```python
from build123d import *

# Parameters (mm, degrees)
SKETCH1_W                      = 76.2
SKETCH1_H                      = 66.04
BOSS_EXTRUDE1_DEPTH            = 20.32
SKETCH2_R                      = 3.749999993
CUT_EXTRUDE1_DEPTH             = 57.15
SKETCH4_W                      = 8
SKETCH4_H                      = 8
CUT_EXTRUDE4_DEPTH             = 5.08
FILLET2_R                      = 2.54
SKETCH5_W                      = 50.8
SKETCH5_H                      = 66.04
BOSS_EXTRUDE2_DEPTH            = 2.54
BOSS_EXTRUDE3_DEPTH            = 25.4
SKETCH3_W                      = 14
SKETCH3_H                      = 7
CUT_EXTRUDE5_DEPTH             = 73.66
CUT_EXTRUDE5_DIRECTION_2_REACH = 29.94
SKETCH7_R                      = 6.35
BOSS_EXTRUDE4_DEPTH            = 30.48


with BuildPart() as part:
    # Sketch1 → Boss-Extrude1 (new body)
    with BuildSketch(Plane.XY):
        with Locations((38.1, 33.02)):
            Rectangle(SKETCH1_W, SKETCH1_H)
    extrude(amount=BOSS_EXTRUDE1_DEPTH)

    # Sketch2 → Cut-Extrude1 (cut)
    with BuildSketch(Plane(origin=(0, 66.04, 0), x_dir=(1, 0, 0), z_dir=(0, 1, 0))):
        with Locations(Location((17.78, -10.16, 0), (0, 0, 270))):  # turned: the seam where the file's is
            Circle(SKETCH2_R)
    extrude(amount=-CUT_EXTRUDE1_DEPTH, mode=Mode.SUBTRACT)

    # Sketch4 → Cut-Extrude4 (cut)
    with BuildSketch(Plane(origin=(0, 0, 0), x_dir=(-1, 0, 0), z_dir=(0, -1, 0))):
        with Locations((-10.16, -10.16)):
            Rectangle(SKETCH4_W, SKETCH4_H)
    extrude(amount=-CUT_EXTRUDE4_DEPTH, mode=Mode.SUBTRACT)

    # Fillet2
    fillet2_edges = [part.edges().sort_by_distance(p)[0] for p in [
        (17.78, 66.04, 6.410000007),
    ]]
    fillet(fillet2_edges, radius=FILLET2_R)

    # Sketch5 → Boss-Extrude2 (add)
    with BuildSketch(Plane(origin=(76.2, 0, 0), x_dir=(0, 0, -1), z_dir=(1, 0, 0))):
        with Locations((0, 33.02)):
            Rectangle(SKETCH5_W, SKETCH5_H)
    extrude(amount=BOSS_EXTRUDE2_DEPTH)

    # Sketch6 → Boss-Extrude3 (add)
    with BuildSketch(Plane(origin=(78.74, 0, 0), x_dir=(0, 0, -1), z_dir=(1, 0, 0))):
        Polygon((-25.4, 0), (-19.631407878, 0), (15.24, 0), (25.4, 0), (25.4, 63.5), (22.86, 63.5), (22.86, 2.54), (-22.86, 2.54), (-22.86, 63.5), (-25.4, 63.5), align=None)
    extrude(amount=BOSS_EXTRUDE3_DEPTH)

    # Sketch3 → Cut-Extrude5 (cut)
    with BuildSketch(Plane(origin=(76.2, 0, 0), x_dir=(0, 0, -1), z_dir=(1, 0, 0))):
        with Locations((-10.16, 8.58)):
            Rectangle(SKETCH3_W, SKETCH3_H)
    extrude(amount=-CUT_EXTRUDE5_DEPTH, mode=Mode.SUBTRACT)

    # Sketch3 → Cut-Extrude5 direction 2 (cut, up to next)
    with BuildSketch(Plane(origin=(76.2, 0, 0), x_dir=(0, 0, -1), z_dir=(1, 0, 0)), mode=Mode.PRIVATE) as cut_extrude5_direction_2_sk1:
        with Locations((-10.16, 8.58)):
            Rectangle(SKETCH3_W, SKETCH3_H)
    cut_extrude5_direction_2_tool1 = extrude(cut_extrude5_direction_2_sk1.sketch, amount=CUT_EXTRUDE5_DIRECTION_2_REACH, mode=Mode.PRIVATE) & part.part
    add(cut_extrude5_direction_2_tool1.solids().sort_by_distance((76.2, 8.58, 10.16))[0], mode=Mode.SUBTRACT)

    # Sketch7 → Boss-Extrude4 (add)
    with BuildSketch(Plane(origin=(0, 0, 0), x_dir=(-1, 0, 0), z_dir=(0, -1, 0))):
        with Locations(Location((-63.5, -10.16, 0), (0, 0, 270))):  # turned: the seam where the file's is
            Circle(SKETCH7_R)
    extrude(amount=BOSS_EXTRUDE4_DEPTH)


solid = part.part
```
Design review of the part built by this model. Coordinates are the model's own, in mm. A direction names the side the tool comes from. Give positions to 0.01 mm unless a question says otherwise; leave off trailing zeros. Write each loop counter-clockwise with the first axis right and the second up, starting at its lowest first coordinate (ties: lowest second). Pieces come first, ordered by that corner, then holes. Notation, with made-up numbers: (77, -23) - (127, -23) arc R24 cw to (127, -10) - close; hole circle Ø9 at (45, 67). An arc over 180 degrees is marked (long way). Return JSON: item names as keys, results as strings. Group by question number.
(1) We need section B-B, the plane x = 63.5. Give the boundary of the cut face in (y, z).
(2) To check wall thickness, follow probe 1 along X at (y, z) = (52.5, 10.16); probe 2 along Z at (x, y) = (58, 48); probe 3 along X at (y, z) = (5, -19). State the ranges of each line that lie inside material, in increasing order.
(3) We need section D-D, the plane x = 17.78. Give the boundary of the cut face in (y, z), then the cut area to 3 significant figures.
(4) We need section C-C, the plane y = 23.5. Give the boundary of the cut face in (x, z).
(5) We need section A-A, the plane z = 10.16. Give the boundary of the cut face in (x, y).
(6) Mouldability with a two-part tool opening along Y and no side actions: class faces 6 (the flat face through (91, 2.54, 0)), 7 (the flat face through (0, 33, 10)), 8 (the flat face through (40, 9, 17.16)) as +Y half, -Y half, draft (parallel to the pull), parting line (faces both ways), or undercut.
(7) Insertion check: pin 1 (10 mm diameter, centred on y = 9, z = -7.5, fed in from +X); pin 2 (5 mm diameter, centred on x = 18.5, z = 5, fed in from -Y); pin 3 (12.5 mm diameter, centred on y = 44.5, z = -13, fed in from -X). Each pin has a flat end and moves straight along its axis. Give the tip position at first contact, or say it passes through.
(8) Machinability: for faces 1 (the flat face through (76.2, 33, -13)), 2 (the flat face through (91, 63.5, -24)), 3 (the flat face through (38, 33, 20.32)), 4 (the flat face through (40, 9, 3.16)), 5 (the flat face through (91, 33, -22.86)), which of the approach directions +Z, -Z, +X, -X, +Y, -Y give a long, thin tool a straight path to every point of the face, cutting with its end or side? Answer none if there is none.
Reported:
{
 "1": {"outline": "(-30.48, 3.81) - (0, 3.81) - (0, 0) - (66.04, 0) - (66.04, 20.32) - (0, 20.32) - (0, 16.51) - (-30.48, 16.51) - close; hole (5.08, 3.16) - (12.08, 3.16) - (12.08, 17.16) - (5.08, 17.16) - close"},
 "2": {"probe 1": "x = 0 to 14.03, 21.53 to 78.74", "probe 2": "z = 0 to 20.32", "probe 3": "x = 76.2 to 78.74"},
 "3": {"outline": "(0, 0) - (66.04, 0) - (66.04, 3.87) arc R2.54 ccw to (63.5, 6.41) - (12.08, 6.41) - (12.08, 3.16) - (5.08, 3.16) - (5.08, 17.16) - (12.08, 17.16) - (12.08, 13.91) - (63.5, 13.91) arc R2.54 ccw to (66.04, 16.45) - (66.04, 20.32) - (0, 20.32) - close", "area": "836 mm2"},
 "4": {"outline": "(0, 0) - (76.2, 0) - (76.2, -25.4) - (104.14, -25.4) - (104.14, -22.86) - (78.74, -22.86) - (78.74, 22.86) - (104.14, 22.86) - (104.14, 25.4) - (76.2, 25.4) - (76.2, 20.32) - (0, 20.32) - close; hole circle Ø7.5 at (17.78, 10.16)"},
 "5": {"outline": "(0, 0) - (6.16, 0) - (6.16, 5.08) - (2.54, 5.08) - (2.54, 12.08) - (14.03, 12.08) - (14.03, 63.5) arc R2.54 ccw to (11.49, 66.04) - (0, 66.04) - close; (14.16, 0) - (57.15, 0) - (57.15, -30.48) - (69.85, -30.48) - (69.85, 0) - (104.14, 0) - (104.14, 2.54) - (78.74, 2.54) - (78.74, 5.08) - (14.16, 5.08) - close; (21.53, 12.08) - (78.74, 12.08) - (78.74, 66.04) - (24.07, 66.04) arc R2.54 ccw to (21.53, 63.5) - close"},
 "6": {"face 6": "+Y half", "face 7": "draft", "face 8": "undercut"},
 "7": {"pin 1": "stops at x = 78.74", "pin 2": "stops at y = 0", "pin 3": "stops at x = 76.2"},
 "8": {"face 1": "-Z, -X, +Y, -Y", "face 2": "+Z, -Z, +X, +Y", "face 3": "+Z, -X, +Y, -Y", "face 4": "+X", "face 5": "+X, +Y"}
}
